Here's how the part is built. I have some questions about the finished solid (model axes, mm). Face numbers are marked on the shaded views. A direction names the side the tool comes from. Coordinates: 2 decimals unless noted, no trailing zeros. Order: outer loops, then holes, each group sorted by start corner. A loop starts at its lowest first (then second) coordinate and runs counter-clockwise, first axis right, second up. Notation, with made-up numbers: (34, 26.25) -> (85, 26.25) arc R10 ccw to (85, 42.25) -> close; hole circle Ø4 at (84.5, -11.5). An arc over 180 degrees is marked (long way). One line per item, written item: value. Start each with the question number.
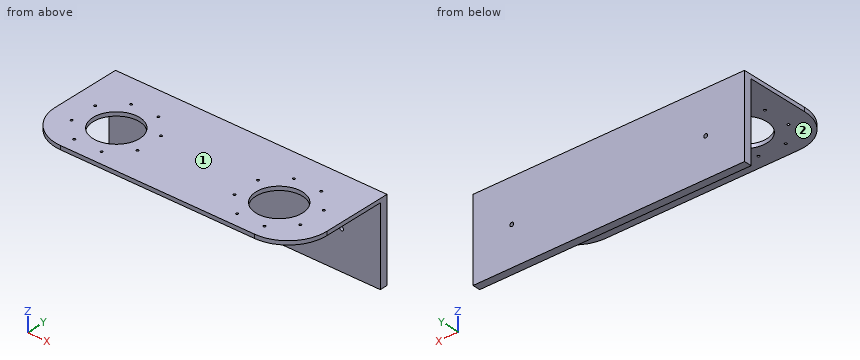
Autodesk Inventor part; units mm, degrees
ref_plane "YZ Plane" through (0, 0, 0) normal (1, 0, 0) x (0, 1, 0)
ref_plane "XZ Plane" through (0, 0, 0) normal (0, 1, 0) x (-1, 0, 0)
ref_plane "XY Plane" through (0, 0, 0) normal (0, 0, 1) x (1, 0, 0)
sketch "スケッチ1" plane through (0, 0, 0) normal (0, 0, 1) x (1, 0, 0)
  line L0 (0, 0) -> (350, 0)
  line L1 (350, 0) -> (350, 140)
  line L2 (350, 140) -> (0, 140)
  circle A0 centre (70, 60) radius 46
  circle A1 centre (280, 60) radius 46
  line L3 (0, 140) -> (0, 0)
  line L4 (70, 60) -> (70, 156.3161)
  line L5 (280, 60) -> (280, 147.5689)
  line L6 (70, 60) -> (45.2011, 119.8698)
  line L7 (280, 60) -> (258.2896, 112.4136)
  circle A2 centre (52.3966, 102.4985) radius 1.5
  circle A3 centre (262.3966, 102.4985) radius 1.5
  circle A4 centre (27.5015, 77.6034) radius 1.5
  circle A5 centre (27.5015, 42.3966) radius 1.5
  circle A6 centre (52.3966, 17.5015) radius 1.5
  circle A7 centre (87.6034, 17.5015) radius 1.5
  circle A8 centre (112.4985, 42.3966) radius 1.5
  circle A9 centre (112.4985, 77.6034) radius 1.5
  circle A10 centre (87.6034, 102.4985) radius 1.5
  circle A11 centre (237.5015, 77.6034) radius 1.5
  circle A12 centre (237.5015, 42.3966) radius 1.5
  circle A13 centre (262.3966, 17.5015) radius 1.5
  circle A14 centre (297.6034, 17.5015) radius 1.5
  circle A15 centre (322.4985, 42.3966) radius 1.5
  circle A16 centre (322.4985, 77.6034) radius 1.5
  circle A17 centre (297.6034, 102.4985) radius 1.5
  circle A18 centre (70, 60) radius 30
  circle A19 centre (280, 60) radius 30
  dimension "d5" = 92
  dimension "d6" = 92
  dimension "d0" = 350
  dimension "d1" = 140
  dimension "d2" = 60
  dimension "d3" = 60
  dimension "d9" = 70
  dimension "d10" = 70
  dimension "d11" = 22.5
  dimension "d12" = 22.5
  dimension "d13" = 3
  dimension "d14" = 3
  dimension "d17" = 360
  dimension "d21" = 360
  dimension "d23" = 60
  dimension "d24" = 60
extrude "押し出し1" add sketch "スケッチ1" along normal blind 5 contours A1 A17 A16 A15 A14 A13 A12 A11 A3 L7 A19 L5 | L5 A19 L7 A3 A1 | A0 A10 A9 A8 A7 A6 A5 A4 A2 L6 A18 L4 | L4 A18 L6 A2 A0 | L3 L2 L1 L0
sketch "スケッチ2" plane through (0, 0, 0) normal (0, 0, -1) x (-1, 0, 0)
  line L0 (-350, 0) -> (-350, 140)
  line L1 (0, 140) -> (-350, 140)
  line L2 (-350, 140) -> (-350, 120)
  line L3 (0, 120) -> (0, 140)
  line L4 (-350, 140) -> (0, 140)
  line L5 (0, 140) -> (0, 130)
  line L6 (0, 130) -> (-350, 130)
  line L7 (-350, 130) -> (-350, 140)
  point P0 (0, 0)
  point P1 (-175, 130)
  dimension "d30" = 10
extrude "押し出し2" add sketch "スケッチ2" along normal blind 100
sketch "スケッチ3" plane through (0, 140, 5) normal (0, 1, 0) x (1, 0, 0)
  circle A0 centre (50, 55) radius 2.5
  circle A1 centre (300, 55) radius 2.5
  line L0 (0, 105) -> (350, 105)
  line L1 (0, 0) -> (0, 105)
  point P0 (0, 5)
  dimension "d31" = 50
  dimension "d32" = 50
  dimension "d33" = 250
  dimension "d34" = 50
  dimension "d35" = 5
  dimension "d36" = 5
extrude "押し出し3" cut sketch "スケッチ3" against normal blind 100
fillet "フィレット2" radius 50 2 edges at (350, 0, 2.5) (0, 0, 2.5)
equation "\"d6\" = d5"
equation "\"d2\" = d3"
equation "\"d10\" = d9"
properties part number "legparts_09"
Q1. For P1, Ø1.8, axis at x = 297.6, y = 102.5, coming from the -Z side; P2, Ø3.5, axis at x = 87.6, y = 17.5, coming from the +Z side; P3, Ø4, axis at x = 237.5, y = 42.4, coming from the -Z side; P4, Ø4, axis at x = 123, z = -20, coming from the -Y side, each with a flat end and sliding along its axis, tell me the tip position at first contact or that it passes through.
Q2. Imagine slicing it at C-C (x = 123.5). Write out the boundary of the cut face in (y, z), plus the area to 3 significant figures.
Q3. For the marked faces 1 and 2, which set-ups out of +Z, -Z, +X, -X, +Y, -Y let a thin tool reach every point of the face, with its end or its side?
Q4. Imagine slicing it at B-B (y = 36.5). Write out the boundary of the cut face in (x, z), plus the area to 3 significant figures.
Q5. I need wall thicknesses on line 1 (Z direction, x = 136.5, y = 80); line 2 (Y direction, x = 74.5, z = -49). Which ranges of each line are inside material? Lowest first, please.
Q6. Imagine slicing it at A-A (x = 70). Write out the boundary of the cut face in (y, z).
Q7. Imagine slicing it at D-D (y = 56). Write out the boundary of the cut face in (x, z), plus the area to 3 significant figures.
Completed:
1. P1: passes through
1. P2: stops at z = 5
1. P3: stops at z = 0
1. P4: stops at y = 130
2. outline: (0, 0) -> (130, 0) -> (130, -100) -> (140, -100) -> (140, 5) -> (0, 5) -> close
2. area: 1,700 mm2
3. face 1: +Z, +X, -X, +Y, -Y
3. face 2: -Z, +X, -X, -Y
4. outline: (1.86, 0) -> (51.35, 0) -> (51.35, 5) -> (1.86, 5) -> close; (88.65, 0) -> (261.35, 0) -> (261.35, 5) -> (88.65, 5) -> close; (298.65, 0) -> (348.14, 0) -> (348.14, 5) -> (298.65, 5) -> close
4. area: 1,360 mm2
5. line 1: z = 0 to 5
5. line 2: y = 130 to 140
6. outline: (0, 0) -> (30, 0) -> (30, 5) -> (0, 5) -> close; (90, 0) -> (130, 0) -> (130, -100) -> (140, -100) -> (140, 5) -> (90, 5) -> close
7. outline: (0, 0) -> (40.27, 0) -> (40.27, 5) -> (0, 5) -> close; (99.73, 0) -> (250.27, 0) -> (250.27, 5) -> (99.73, 5) -> close; (309.73, 0) -> (350, 0) -> (350, 5) -> (309.73, 5) -> close
7. area: 1,160 mm2
